from build123d import *

# Parameters (mm, degrees)
PAD_DEPTH       = 16
SKETCH001_W     = 112
SKETCH001_H     = 1.5
SKETCH001_W_2   = 16
SKETCH001_H_2   = 7.5
POCKET_DEPTH    = 15.5
SKETCH002_W     = 2
SKETCH002_H     = 12.5
SKETCH002_H_2   = 4
SKETCH002_H_3   = 6.5
POCKET001_DEPTH = 5


with BuildPart() as part:
    # Sketch → Pad (new body)
    with BuildSketch(Plane.XY):
        Polygon((-60, 7.5), (60, 7.5), (60, -7.5), (-60, -7.5), (-78, -7.5), (-78, 7.5), align=None)
    extrude(amount=PAD_DEPTH)

    # Sketch001 → Pocket (cut)
    with BuildSketch(Plane.XY):
        with Locations((0, 5.75)):
            Rectangle(SKETCH001_W, SKETCH001_H)
        with Locations((9.5, 0.25)):
            Rectangle(SKETCH001_W_2, SKETCH001_H_2)
        with Locations((-13, 0.25)):
            Rectangle(SKETCH001_W_2, SKETCH001_H_2)
        with Locations((-65, 2.75)):
            Rectangle(SKETCH001_W_2, SKETCH001_H_2)
    extrude(amount=POCKET_DEPTH, mode=Mode.SUBTRACT)

    # Sketch002 → Pocket001 (cut)
    with BuildSketch(Plane.XY):
        with Locations((0, -1.25)):
            Rectangle(SKETCH002_W, SKETCH002_H)
        with Locations((-13, -5.5)):
            Rectangle(SKETCH002_W, SKETCH002_H_2)
        with Locations((9.5, -5.5)):
            Rectangle(SKETCH002_W, SKETCH002_H_2)
        with Locations((-65, -4.25)):
            Rectangle(SKETCH002_W, SKETCH002_H_3)
    extrude(amount=POCKET001_DEPTH, mode=Mode.SUBTRACT)


solid = part.part
Geometry: final body of the model. Coordinates: model frame, mm. A direction names the side the tool comes from. Round coordinates to 2 decimals unless told otherwise and drop trailing zeros. Order: outer loops, then holes, each group sorted by start corner. A loop starts at its lowest first (then second) coordinate and runs counter-clockwise, first axis right, second up.
Q1. Section C-C, the plane y = -2.25. Output: boundary loops of the cut face in (x, z).
Result sheet:
outline: (-78, 0) - (-66, 0) - (-66, 5) - (-64, 5) - (-64, 0) - (-21, 0) - (-21, 15.5) - (-5, 15.5) - (-5, 0) - (-1, 0) - (-1, 5) - (1, 5) - (1, 0) - (1.5, 0) - (1.5, 15.5) - (17.5, 15.5) - (17.5, 0) - (60, 0) - (60, 16) - (-78, 16) - close
Q2. Access query for faces 5 (the face through (10.5, -6, 2)), 6 (the face through (-65, -1, 8)), 7 (the face through (-8, 0, 16)). Directions: +Z, -Z, +X, -X, +Y, -Y. A direction counts if a zero-diameter tool reaches every point of the face in a straight line with its end or side. Return the directions, or none.
Result sheet:
face 5: -Z, -Y
face 6: -Z
face 7: +Z, +X, -X, +Y, -Y
Q3. Section D-D, the plane x = -47. Output: boundary loops of the cut face in (y, z).
Result sheet:
outline: (-7.5, 0) - (5, 0) - (5, 15.5) - (6.5, 15.5) - (6.5, 0) - (7.5, 0) - (7.5, 16) - (-7.5, 16) - close
Q4. Mould query, pull axis Y, two halves, no side actions, for faces 1 (the face through (-73, 3, 8)), 2 (the face through (17.5, 0, 8)), 3 (the face through (-8, 7.5, 8)), 4 (the face through (-64, -4, 2)). Classes: released by +Y, released by -Y, zero draft, split by the parting line, or undercut.
Result sheet:
face 1: undercut
face 2: undercut
face 3: released by +Y
face 4: zero draft
Q5. Section A-A, the plane x = -9. Output: boundary loops of the cut face in (y, z), and give its area (4 significant figures).
Result sheet:
outline: (-7.5, 0) - (-3.5, 0) - (-3.5, 15.5) - (4, 15.5) - (4, 0) - (5, 0) - (5, 15.5) - (6.5, 15.5) - (6.5, 0) - (7.5, 0) - (7.5, 16) - (-7.5, 16) - close
area: 100.5 mm2
Q6. Material intervals for probe 1 along X at (y, z) = (-0.5, 14.5); probe 2 along Y at (x, z) = (-20, 12.75); probe 3 along X at (y, z) = (-2, 6.25), sorted ascending.
Result sheet:
probe 1: x = -78 to -73, -57 to -21, -5 to 1.5, 17.5 to 60
probe 2: y = -7.5 to -3.5, 4 to 5, 6.5 to 7.5
probe 3: x = -78 to -21, -5 to 1.5, 17.5 to 60
Q7. Section B-B, the plane z = 7.75. Output: boundary loops of the cut face in (x, y).
Result sheet:
outline: (-78, -7.5) - (60, -7.5) - (60, 7.5) - (-78, 7.5) - close; hole (-73, -1) - (-57, -1) - (-57, 6.5) - (-73, 6.5) - close; hole (-56, 5) - (56, 5) - (56, 6.5) - (-56, 6.5) - close; hole (-21, -3.5) - (-5, -3.5) - (-5, 4) - (-21, 4) - close; hole (1.5, -3.5) - (17.5, -3.5) - (17.5, 4) - (1.5, 4) - close
